```python
from build123d import *

# Parameters (mm, degrees)
F1_DEPTH  = 6
F3_DEPTH  = 20
F5_DEPTH  = 6
F7_DEPTH  = 40
F9_DEPTH  = 40
F10_R     = 2.25
F11_DEPTH = 8
F12_R     = 2.25
F13_DEPTH = 8
F14_R     = 2.25
F15_DEPTH = 8
F16_R     = 2.25
F17_DEPTH = 8
F18_R     = 3.75
F19_DEPTH = 3
F20_R     = 3.75
F21_DEPTH = 3
F22_R     = 3.75
F23_DEPTH = 3
F24_R     = 3.75
F25_DEPTH = 3
F26_SIZE  = 3


with BuildPart() as f1:
    # F0 (on Top) → F1 (new body)
    with BuildSketch(Plane.XY):
        Polygon((26, 40), (3.85853, 40), (-6, 40), (-6, -6), (60, -6), (60, 26), (26, 26), align=None)
    extrude(amount=F1_DEPTH)

    # F2 (on face) → F3 (join)
    with BuildSketch(Plane.XY.offset(6)):
        Polygon((0, 40), (-6, 40), (-6, -6), (60, -6), (60, 0), (0, 0), align=None)
    extrude(amount=F3_DEPTH)

    # F4 (on face) → F5 (join)
    with BuildSketch(Plane.XY.offset(26)):
        Polygon((-6, 40), (-6, -6), (60, -6), (60, 26), (26, 26), (26, 40), align=None)
    extrude(amount=F5_DEPTH)

    # F6 (on face) → F7 (join)
    with BuildSketch(Plane.YZ.offset(60)):
        Polygon((15.71, 26), (13, 26), (10.29, 26), (10.29, 24), (15.71, 24), align=None)
        Polygon((10.29, 6), (13, 6), (15.71, 6), (15.71, 8), (10.29, 8), align=None)
        Polygon((0, 18.71), (0, 16), (0, 13.29), (2, 13.29), (2, 18.71), align=None)
    extrude(amount=-F7_DEPTH)

    # F8 (on face) → F9 (join)
    with BuildSketch(Plane(origin=(0, 40, 0), x_dir=(-1, 0, 0), z_dir=(0, 1, 0))):
        Polygon((0, 13.29), (0, 16), (0, 18.71), (-2, 18.71), (-2, 13.29), align=None)
        Polygon((-7.29, 26), (-10, 26), (-12.71, 26), (-12.71, 24), (-7.29, 24), align=None)
        Polygon((-12.71, 6), (-10, 6), (-7.29, 6), (-7.29, 8), (-12.71, 8), align=None)
    extrude(amount=-F9_DEPTH)

    # F10 (on face) → F11 (cut, through all)
    with BuildSketch(Plane(origin=(0, 0, 0), x_dir=(1, 0, 0), z_dir=(0, 0, -1))):
        with Locations((50, -13)):
            Circle(F10_R)
        with Locations((10, -30)):
            Circle(F10_R)
    extrude(amount=-F11_DEPTH, mode=Mode.SUBTRACT)

    # F12 (on face) → F13 (cut, through all)
    with BuildSketch(Plane.XY.offset(32)):
        with Locations((10, 10)):
            Circle(F12_R)
        with Locations((30, 13)):
            Circle(F12_R)
    extrude(amount=-F13_DEPTH, mode=Mode.SUBTRACT)

    # F14 (on face) → F15 (cut, through all)
    with BuildSketch(Plane.XZ.offset(6)):
        with Locations((40, 16)):
            Circle(F14_R)
    extrude(amount=-F15_DEPTH, mode=Mode.SUBTRACT)

    # F16 (on face) → F17 (cut, through all)
    with BuildSketch(Plane(origin=(-6, 0, 0), x_dir=(0, -1, 0), z_dir=(-1, 0, 0))):
        with Locations((-20, 16)):
            Circle(F16_R)
    extrude(amount=-F17_DEPTH, mode=Mode.SUBTRACT)

    # F18 (on face) → F19 (cut)
    with BuildSketch(Plane.XY.offset(32)):
        with Locations((10, 10)):
            Circle(F18_R)
        with Locations((30, 13)):
            Circle(F18_R)
    extrude(amount=-F19_DEPTH, mode=Mode.SUBTRACT)

    # F20 (on face) → F21 (cut)
    with BuildSketch(Plane(origin=(-6, 0, 0), x_dir=(0, -1, 0), z_dir=(-1, 0, 0))):
        with Locations((-20, 16)):
            Circle(F20_R)
    extrude(amount=-F21_DEPTH, mode=Mode.SUBTRACT)

    # F22 (on face) → F23 (cut)
    with BuildSketch(Plane(origin=(0, 0, 0), x_dir=(1, 0, 0), z_dir=(0, 0, -1))):
        with Locations((10, -30)):
            Circle(F22_R)
        with Locations((50, -13)):
            Circle(F22_R)
    extrude(amount=-F23_DEPTH, mode=Mode.SUBTRACT)

    # F24 (on face) → F25 (cut)
    with BuildSketch(Plane.XZ.offset(6)):
        with Locations((40, 16)):
            Circle(F24_R)
    extrude(amount=-F25_DEPTH, mode=Mode.SUBTRACT)

    # F26
    f26_edges = [f1.edges().sort_by_distance(p)[0] for p in [
        (27, -6, 0),
        (43, 26, 0),
        (26, 33, 0),
        (10, 40, 0),
        (-6, 17, 0),
        (-6, -6, 16),
        (27, -6, 32),
        (-6, 17, 32),
        (10, 40, 32),
        (26, 33, 32),
        (43, 26, 32),
        (60, 10, 32),
        (60, 10, 0),
        (-6, 40, 16),
        (60, -6, 16),
    ]]
    chamfer(f26_edges, length=F26_SIZE)


solid = f1.part
```
Geometry: final body of the model. Coordinates: model frame, mm. A direction names the side the tool comes from. Round coordinates to 2 decimals unless told otherwise and drop trailing zeros. Loops run counter-clockwise (first coordinate to the right, second up) from the corner with the lowest first, then second, coordinate; pieces in that order, holes last. Notation, with made-up numbers: (87.25, 23.5) -> (132.25, 23.5) arc R27 ccw to (132.25, 40.5) -> close; hole circle Ø4 at (-8.5, 32.25). An arc over 180 degrees is marked (long way). Write each question's results on one line, items separated by ' | '.
Item 1: Set-up query: faces 5 (the face through (43, 26, 4)), 6 (the face through (1, 20, 18.71)), 7 (the face through (8.34, 11.52, 26.54)), 8 (the face through (52, 15, 3)), 9 (the face through (20, 1, 16)). Return all of +Z, -Z, +X, -X, +Y, -Y with unobstructed straight access to the full face (end or side cutting, diameter ignored); none if empty.
Answers below:
face 5: +Z, -Z, +X, +Y | face 6: +X, +Y | face 7: +Z | face 8: -Z | face 9: +Y
Item 2: Line query: probe 1 along X at (y, z) = (30, 6.15); probe 2 along Z at (x, y) = (36, 0.5); probe 3 along Y at (x, z) = (10, 26). Output: solid intervals per line, ascending. Write a range as [from, to].
Answers below:
probe 1: x = [-6, 0], [7.29, 7.75], [12.25, 12.71] | probe 2: z = [0, 6], [13.29, 18.71], [26, 32] | probe 3: y = [-6, 7.75], [12.25, 40]
Item 3: Pull-direction query (Z, two-part tool) for faces 1 (the face through (10, 20, 8)), 2 (the face through (7.236, 12.534, 30.521)), 3 (the face through (-4, -4, 2)), 4 (the face through (12, 8, 29)); classes: pulls with the +Z half, pulls with the -Z half, needs draft (parallel to the pull), parting line crosses it, or undercut.
Answers below:
face 1: undercut | face 2: needs draft | face 3: pulls with the -Z half | face 4: pulls with the +Z half
Item 4: Pin query (flat end, axial travel): pin 1 Ø2.5 at (y, z) = (36, 4) entering from +X; pin 2 Ø1.6 at (y, z) = (17, 16) entering from +X; pin 3 Ø2 at (x, z) = (3.5, 15.5) entering from +Y. Return the tip coordinate at first contact, or that it passes through.
Answers below:
pin 1: stops at x = 26 | pin 2: stops at x = 2 | pin 3: stops at y = 0
Item 5: Cut plane D-D on z = 16. Return the cut outline in (x, y).
Answers below:
outline: (-6, -3) -> (-3, -6) -> (36.25, -6) -> (36.25, -3) -> (37.75, -3) -> (37.75, 2) -> (20, 2) -> (20, 0) -> (2, 0) -> (2, 17.75) -> (-3, 17.75) -> (-3, 16.25) -> (-6, 16.25) -> close; (-6, 23.75) -> (-3, 23.75) -> (-3, 22.25) -> (2, 22.25) -> (2, 40) -> (-3, 40) -> (-6, 37) -> close; (42.25, -3) -> (43.75, -3) -> (43.75, -6) -> (57, -6) -> (60, -3) -> (60, 2) -> (42.25, 2) -> close
Item 6: Cut plane C-C on z = 27. Return the cut outline in (x, y), and give its area (3 significant figures).
Answers below:
outline: (-6, -3) -> (-3, -6) -> (57, -6) -> (60, -3) -> (60, 26) -> (26, 26) -> (26, 40) -> (-3, 40) -> (-6, 37) -> close; hole circle Ø4.5 at (10, 10); hole circle Ø4.5 at (30, 13) | area: 2,510 mm²
